from build123d import *

# Parameters (mm, degrees)
F0_R     = 66.408599
F0_R_2   = 63.646322
F1_DEPTH = 25
F2_T     = -2.5


with BuildPart() as f1:
    # F0 (on Right) → F1 (new body)
    with BuildSketch(Plane.YZ):
        Circle(F0_R)
        Circle(F0_R_2, mode=Mode.SUBTRACT)
    extrude(amount=F1_DEPTH)

    # F2
    f2_openings = [f1.faces().sort_by_distance(p)[0] for p in [
        (12.5, -63.646322, 0),
    ]]
    offset(amount=F2_T, openings=f2_openings)


solid = f1.part
Verification items for the finished model (mm, model axes). Coordinates: 2 decimals unless noted, no trailing zeros. Order: outer loops, then holes, each group sorted by start corner. A loop starts at its lowest first (then second) coordinate and runs counter-clockwise, first axis right, second up. Notation, with made-up numbers: M 46,-10 L 65,-10 A22 cw 65,22 Z; hole C -7,28.5 d8. An arc over 180 degrees is marked long. One line per item, written item: value. Start each with the question number.
Item 1: Sectioned sample at C-C (x = 12.25). Enter the section's corners in (y, z), then the cut area to 3 significant figures.
Item 2: Mould release check, pull along X, two halves, no side actions. Record for faces 1 (the cylindrical face through (12.32, -52.7, -40.41)), 2 (the cylindrical face through (12.36, -50.716, -38.887)), 3 (the flat face through (25, 34, -54)): released by +X, released by -X, zero draft, split by the parting line, or undercut.
Item 3: Sectioned sample at A-A (y = 0). Enter the section's corners in (x, z), then the cut area to 3 significant figures.
Item 4: Scan lines: probe 1 along Z at (x, y) = (23.95, 0); probe 2 along Y at (x, z) = (4.5, 5.5); probe 3 along Z at (x, y) = (13.75, -45.5). Record each from-to range of solid material in increasing order.
Item 5: Sectioned sample at B-B (z = -49.5). Enter the section's corners in (x, y).
Item 6: Gauge pin test, flat ends, axial feed: pin 1 (8 mm diameter, centred on x = 13, y = -48.5, fed in from -Z); pin 2 (4 mm diameter, centred on x = 8.5, y = -24.5, fed in from +Z); pin 3 (1 mm diameter, centred on x = 5, y = -45, fed in from +Z). Record the tip position at first contact, or that the pin passes through.
Conclusion:
1. outline: C 0,0 d132.82; hole C 0,0 d127.82
1. area: 1,020 mm^2
2. face 1: zero draft
2. face 2: undercut
2. face 3: released by +X
3. outline: M 0,-66.41 L 25,-66.41 L 25,-63.65 L 22.5,-63.65 L 22.5,-63.91 L 2.5,-63.91 L 2.5,-63.65 L 0,-63.65 Z; M 0,63.65 L 2.5,63.65 L 2.5,63.91 L 22.5,63.91 L 22.5,63.65 L 25,63.65 L 25,66.41 L 0,66.41 Z
3. area: 128 mm^2
4. probe 1: z = -66.41 to -63.65, 63.65 to 66.41
4. probe 2: y = -66.18 to -63.67, 63.67 to 66.18
4. probe 3: z = -48.37 to -44.88, 44.88 to 48.37
5. outline: M 0,-44.27 L 25,-44.27 L 25,-40.01 L 22.5,-40.01 L 22.5,-40.42 L 2.5,-40.42 L 2.5,-40.01 L 0,-40.01 Z; M 0,40.01 L 2.5,40.01 L 2.5,40.42 L 22.5,40.42 L 22.5,40.01 L 25,40.01 L 25,44.27 L 0,44.27 Z
6. pin 1: stops at z = -49.29
6. pin 2: stops at z = 62.48
6. pin 3: stops at z = 49.29
